Geometry: final body of the model. Coordinates: model frame, mm. Face numbers are marked on the shaded views. Coordinates: 2 decimals unless noted, no trailing zeros. Loops run counter-clockwise (first coordinate to the right, second up) from the corner with the lowest first, then second, coordinate; pieces in that order, holes last. Notation, with made-up numbers: M 30,35 L 58,35 A16 ccw 58,51 Z; hole C -27.75,-21.5 d1. An arc over 180 degrees is marked long. Write item = value, one per line. Start each with the question number.
```python
from build123d import *

# Parameters (mm, degrees)
F0_R            = 63.5
F0_R_2          = 15.875
F1_DEPTH        = 25.4
F2_R            = 6.35
F3_DEPTH        = 25.4
F3_COPIES_COUNT = 5


# Not quite as in the source:
# - a pattern or mirror of a feature is missing from the dataset's text; its kind, count and spacing are read off the source's solid


with BuildPart() as f1:
    # F0 (on Front) → F1 (new body)
    with BuildSketch(Plane.XZ):
        Circle(F0_R)
        Circle(F0_R_2, mode=Mode.SUBTRACT)
    extrude(amount=F1_DEPTH)

    # F2 (on face) → F3 (cut, through all)
    with BuildSketch(Plane.XZ.offset(25.4)):
        with Locations((0, 50.8)):
            Circle(F2_R)
        with Locations((0, 31.75)):
            Circle(F2_R)
    f3 = extrude(amount=-F3_DEPTH, mode=Mode.SUBTRACT)

    # F3_copies: F3 ×5 about axis
    f3_copies_axis = Axis((0, 0, 0), (0, 1, 0))
    for i in range(1, F3_COPIES_COUNT):
        add(f3.rotate(f3_copies_axis, i * 360 / F3_COPIES_COUNT), mode=Mode.SUBTRACT)


solid = f1.part
```
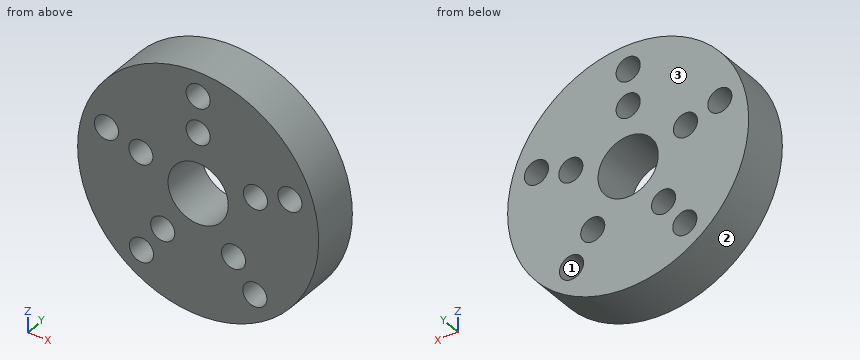
Item 1: Section query C-C (y = -18.5). Count the separate pieces of the cut face and the enclosed holes in it, plus the area to 3 significant figures.
Item 2: Section query A-A (z = 50.8). Return the cut outline in (x, y), plus the area to 3 significant figures.
Item 3: Pull-direction query (Z, two-part tool) for the marked faces 1, 2 and 3; classes: released by +Z, released by -Z, zero draft, split by the parting line, or undercut.
Item 4: Section query D-D (z = 0). Return the cut outline in (x, y) (3 decimals).
Item 5: Line query: line 1 (X direction, y = -19.5, z = -28); line 2 (Z direction, x = -54, y = -17); line 3 (X direction, y = -23, z = 18.5). Output: solid intervals per line, ascending. Write a range as from..to.
Item 6: First-contact query: pin 1 (7.5 mm diameter, centred on x = -48.31, z = 15.7, fed in from +Y); pin 2 (8 mm diameter, centred on x = -3.5, y = -17.5, fed in from -Z); pin 3 (12 mm diameter, centred on x = -46.5, y = -12, fed in from -Z); pin 4 (1 mm diameter, centred on y = -18, z = 14, fed in from -X). Flat tips, straight axial feed; report the tip coordinate or a pass-through.
Item 7: Section query B-B (x = 3). Return the cut outline in (y, z).
Verdict:
q1.separate_pieces = 1
q1.enclosed_holes = 11
q1.area = 10,600 mm2
q2.outline = M -38.1,-25.4 L -6.35,-25.4 L -6.35,0 L -38.1,0 Z; M 6.35,-25.4 L 38.1,-25.4 L 38.1,0 L 6.35,0 Z
q2.area = 1,610 mm2
q3.face_1 = undercut
q3.face_2 = split by the parting line
q3.face_3 = zero draft
q4.outline = M -63.5,-25.4 L -15.875,-25.4 L -15.875,0 L -63.5,0 Z; M 15.875,-25.4 L 63.5,-25.4 L 63.5,0 L 15.875,0 Z
q5.line_1 = -56.99..-24.58, -12.75..12.75, 24.58..56.99
q5.line_2 = -33.41..12.87, 18.52..33.41
q5.line_3 = -60.75..-54.01, -42.62..42.62, 54.01..60.75
q6.pin_1 = through
q6.pin_2 = -63.5
q6.pin_3 = -48.91
q6.pin_4 = -62.05
q7.outline = M -25.4,-63.43 L 0,-63.43 L 0,-15.59 L -25.4,-15.59 Z; M -25.4,15.59 L 0,15.59 L 0,26.15 L -25.4,26.15 Z; M -25.4,37.35 L 0,37.35 L 0,45.2 L -25.4,45.2 Z; M -25.4,56.4 L 0,56.4 L 0,63.43 L -25.4,63.43 Z
